The listing builds one solid part. Answer for the finished solid, in the listing's coordinates (mm). Face numbers are marked on the shaded views. A direction names the side the tool comes from. Coordinates: 2 decimals unless noted, no trailing zeros. Loops run counter-clockwise (first coordinate to the right, second up) from the corner with the lowest first, then second, coordinate; pieces in that order, holes last. Notation, with made-up numbers: M -13,19 L 29,19 A14 cw 29,29 Z; hole C 53,-17 d2. An arc over 180 degrees is marked long. Answer as CSV lines item,"result". Start each with the question number.
```python
from build123d import *

# Parameters (mm, degrees)
EXTRUDE_1_DEPTH     = 37.9
CUT_EXTRUDE_1_REACH = 70.771
SKETCH_2_R          = 1.5
FILLET_1_R          = 1


with BuildPart() as part:
    # 草图1 → 凸台-拉伸1 (new body)
    with BuildSketch(Plane.XY):
        with BuildLine():
            Line((0, 0), (0, -7.2))
            Line((0, -7.2), (19.37157627, -7.263562842))
            ThreePointArc((19.37157627, -7.263562842), (33, -21.5), (19.37157627, -35.736437158))
            Line((19.37157627, -35.736437158), (0, -35.8))
            Line((0, -35.8), (0, -43))
            Line((0, -43), (3, -43))
            Line((3, -43), (3, -37.5))
            Line((3, -37.5), (6, -37.5))
            Line((6, -37.5), (12.56027856, -39.727721978))
            ThreePointArc((12.56027856, -39.727721978), (38, -21.5), (12.56027856, -3.272278022))
            Line((12.56027856, -3.272278022), (6, -5.5))
            Line((6, -5.5), (3, -5.5))
            Line((3, -5.5), (3, 0))
            Line((3, 0), (0, 0))
        make_face()
    extrude(amount=EXTRUDE_1_DEPTH)

    # 草图2 → 切除-拉伸1 (cut, up to next)
    with BuildSketch(Plane.ZY, mode=Mode.PRIVATE) as cut_extrude_1_sk1:
        with Locations((3, -2.3)):
            Circle(SKETCH_2_R)
    cut_extrude_1_tool1 = extrude(cut_extrude_1_sk1.sketch, amount=-CUT_EXTRUDE_1_REACH, mode=Mode.PRIVATE) & part.part
    # 草图2 → 切除-拉伸1 (cut, up to next)
    with BuildSketch(Plane.ZY, mode=Mode.PRIVATE) as cut_extrude_1_sk2:
        with Locations(Location((34.9, -2.3, 0), (0, 0, 270))):
            Circle(SKETCH_2_R)
    cut_extrude_1_tool2 = extrude(cut_extrude_1_sk2.sketch, amount=-CUT_EXTRUDE_1_REACH, mode=Mode.PRIVATE) & part.part
    # 草图2 → 切除-拉伸1 (cut, up to next)
    with BuildSketch(Plane.ZY, mode=Mode.PRIVATE) as cut_extrude_1_sk3:
        with Locations(Location((3, -40.7, 0), (0, 0, 270))):
            Circle(SKETCH_2_R)
    cut_extrude_1_tool3 = extrude(cut_extrude_1_sk3.sketch, amount=-CUT_EXTRUDE_1_REACH, mode=Mode.PRIVATE) & part.part
    # 草图2 → 切除-拉伸1 (cut, up to next)
    with BuildSketch(Plane.ZY, mode=Mode.PRIVATE) as cut_extrude_1_sk4:
        with Locations((34.9, -40.7)):
            Circle(SKETCH_2_R)
    cut_extrude_1_tool4 = extrude(cut_extrude_1_sk4.sketch, amount=-CUT_EXTRUDE_1_REACH, mode=Mode.PRIVATE) & part.part
    add(cut_extrude_1_tool1.solids().sort_by_distance((0, -2.3, 3))[0], mode=Mode.SUBTRACT)
    add(cut_extrude_1_tool2.solids().sort_by_distance((0, -2.3, 34.9))[0], mode=Mode.SUBTRACT)
    add(cut_extrude_1_tool3.solids().sort_by_distance((0, -40.7, 3))[0], mode=Mode.SUBTRACT)
    add(cut_extrude_1_tool4.solids().sort_by_distance((0, -40.7, 34.9))[0], mode=Mode.SUBTRACT)

    # 圆角1
    fillet_1_edges = [part.edges().sort_by_distance(p)[0] for p in [
        (1.5, -43, 0),
        (1.5, 0, 0),
        (1.5, -43, 37.9),
        (1.5, 0, 37.9),
    ]]
    fillet(fillet_1_edges, radius=FILLET_1_R)


solid = part.part
```
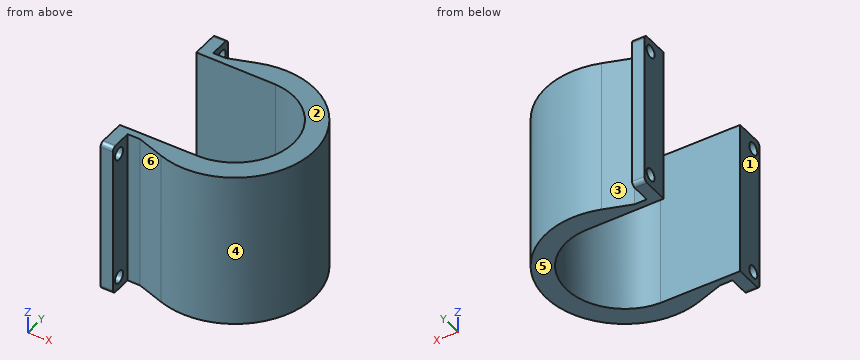
Item 1: Section D-D on x = 20.5 is taken. Determine the outline of the cut face in (y, z), then the cut area to 3 significant figures.
Item 2: For the marked faces 5 and 6, determine the directions among +Z, -Z, +X, -X, +Y, -Y from which every point of the face is accessible in a straight line to the end or side of a thin tool.
Item 3: Section C-C on y = -21.5 is taken. Determine the outline of the cut face in (x, z).
Item 4: Consider line 1 (Z direction, x = 2, y = -2); line 2 (Y direction, x = 2, z = 34); line 3 (Z direction, x = 1, y = -40). Determine where each line is inside the solid, lowest interval first.
Item 5: For a pull along X with two mould halves and no side action, classify the marked faces 1, 2, 3 and 4 as pulls with the +X half, pulls with the -X half, needs draft (parallel to the pull), parting line crosses it, or undercut.
Item 6: Section A-A on z = 34.9 is taken. Determine the outline of the cut face in (x, y).
Item 7: Each of these flat-tipped pins is pushed along its axis until it touches: P1, Ø12, axis at y = -32.5, z = 9.5, coming from the +X side; P2, Ø12, axis at x = 10, z = 16.5, coming from the +Y side; P3, Ø3.5, axis at y = -40.7, z = 3, coming from the +X side; P4, Ø8, axis at x = 5, y = -32.5, coming from the -Z side. Where does it stop, or does it pass through?
Item 8: Section B-B on x = 28.5 is taken. Determine the outline of the cut face in (y, z), then the cut area to 3 significant figures.
Results are:
1,outline,"M -40.67,0 L -35.64,0 L -35.64,37.9 L -40.67,37.9 Z; M -7.36,0 L -2.33,0 L -2.33,37.9 L -7.36,37.9 Z"
1,area,"381 mm²"
2,face 5,"-Z, +X, -X, +Y, -Y"
2,face 6,"+Z, -Z, -Y"
3,outline,"M 33,0 L 38,0 L 38,37.9 L 33,37.9 Z"
4,line 1,"0 to 1.53, 4.47 to 33.43, 36.37 to 37.9"
4,line 2,"-43 to -41.9, -39.5 to -35.79, -7.21 to -3.5, -1.1 to 0"
4,line 3,"0 to 1.67, 4.33 to 33.57, 36.23 to 37.9"
5,face 1,"pulls with the -X half"
5,face 2,"needs draft"
5,face 3,"undercut"
5,face 4,"undercut"
6,outline,"M 0,-43 L 3,-43 L 3,-42.2 L 0,-42.2 Z; M 0,-39.2 L 3,-39.2 L 3,-37.5 L 6,-37.5 L 12.56,-39.73 A19.25 ccw long 12.56,-3.27 L 6,-5.5 L 3,-5.5 L 3,-3.8 L 0,-3.8 L 0,-7.2 L 19.37,-7.26 A14.25 cw 19.37,-35.74 L 0,-35.8 Z; M 0,-0.8 L 3,-0.8 L 3,0 L 0,0 Z"
7,P1,"x = 37.34"
7,P2,"y = -2.45"
7,P3,"x = 26.88"
7,P4,"z = 0"
8,outline,"M -38.1,0 L -31.89,0 L -31.89,37.9 L -38.1,37.9 Z; M -11.11,0 L -4.9,0 L -4.9,37.9 L -11.11,37.9 Z"
8,area,"470 mm²"
